```python
from build123d import *

# Parameters (mm, degrees)
F0_W      = 157
F0_H      = 90
F1_DEPTH  = 83
F3_DEPTH  = 90
F5_DEPTH  = 557
F6_R      = 22
F7_DEPTH  = 25
F7_FACE_R = 22
F8_DEPTH  = 185


with BuildPart() as f1:
    # F0 (on Top) → F1 (new body)
    with BuildSketch(Plane.XY):
        Rectangle(F0_W, F0_H)
    extrude(amount=F1_DEPTH)

    # F2 (on face) → F3 (join, through all)
    with BuildSketch(Plane.XZ.offset(45)):
        with BuildLine():
            Line((-78.5, 0), (-78.5, 83))
            ThreePointArc((-78.5, 83), (-89.175701, 41.5), (-78.5, 0))
        make_face()
        with BuildLine():
            ThreePointArc((78.5, 0), (89.175701, 41.5), (78.5, 83))
            Line((78.5, 83), (78.5, 0))
        make_face()
    extrude(amount=-F3_DEPTH)

    # F4 (on face) → F5 (cut)
    with BuildSketch(Plane.XZ.offset(45)):
        Polygon((-56.5, 0), (-4, 0), (48.5, 0), (48.5, 22), (-56.5, 22), align=None)
    extrude(amount=-F5_DEPTH, mode=Mode.SUBTRACT)

    # F6 (on face) → F7 (cut)
    with BuildSketch(Plane.XY.offset(83)):
        with BuildLine():
            ThreePointArc((0, -35), (24.748737, -24.748737), (35, 0))
            ThreePointArc((35, 0), (24.748737, 24.748737), (0, 35))
            ThreePointArc((0, 35), (-35, 0), (0, -35))
        make_face()
        Circle(F6_R, mode=Mode.SUBTRACT)
        with BuildLine():
            ThreePointArc((0, 35), (24.748737, 24.748737), (35, 0))
            ThreePointArc((35, 0), (24.748737, -24.748737), (0, -35))
            Line((0, -35), (78.5, -35))
            Line((78.5, -35), (78.5, 35))
            Line((78.5, 35), (0, 35))
        make_face()
        Polygon((93.384914, 35), (78.5, 35), (78.5, -35), (92.262775, -35), (93.384914, -35.542417), align=None)
    extrude(amount=-F7_DEPTH, mode=Mode.SUBTRACT)

    # F7_face (on face) → F8 (cut)
    with BuildSketch(Plane.XY.offset(83)):
        Circle(F7_FACE_R)
    extrude(amount=-F8_DEPTH, mode=Mode.SUBTRACT)


solid = f1.part
```
Geometry: final body of the model. Coordinates: model frame, mm. A direction names the side the tool comes from. Coordinates: 2 decimals unless noted, no trailing zeros. Order: outer loops, then holes, each group sorted by start corner. A loop starts at its lowest first (then second) coordinate and runs counter-clockwise, first axis right, second up. Notation, with made-up numbers: (69.25, 60.5) -> (87.25, 60.5) arc R27 ccw to (87.25, 96.5) -> close; hole circle Ø6 at (-21, -38.75). An arc over 180 degrees is marked (long way). Write item = value, one per line.
(1) Line query: line 1 (Y direction, x = 15, z = 66); line 2 (Y direction, x = 0, z = 47); line 3 (Z direction, x = -16.5, y = -20.5). Output: solid intervals per line, ascending.
Solved:
line_1 = -45 to -35, 35 to 45
line_2 = -45 to -22, 22 to 45
line_3 = 22 to 58
(2) Pin query (flat end, axial travel): pin 1 Ø5 at (x, y) = (21.5, -30.5) entering from +Z; pin 2 Ø8 at (y, z) = (29, 19) entering from -X; pin 3 Ø6.5 at (y, z) = (-5.5, 7.5) entering from +X. Return the tip coordinate at first contact, or that it passes through.
Solved:
pin_1 = 58
pin_2 = -87.16
pin_3 = 83.49
(3) Cut plane D-D on x = -2. Return loops of the section in (y, z).
Solved:
outline = (-45, 22) -> (-21.91, 22) -> (-21.91, 58) -> (-34.94, 58) -> (-34.94, 83) -> (-45, 83) -> close; (21.91, 22) -> (45, 22) -> (45, 83) -> (34.94, 83) -> (34.94, 58) -> (21.91, 58) -> close
(4) Cut plane C-C on x = 53.5. Return loops of the section in (y, z).
Solved:
outline = (-45, 0) -> (45, 0) -> (45, 83) -> (35, 83) -> (35, 58) -> (-35, 58) -> (-35, 83) -> (-45, 83) -> close
(5) Cut plane B-B on z = 10. Return loops of the section in (x, y).
Solved:
outline = (-83.2, -45) -> (-56.5, -45) -> (-56.5, 45) -> (-83.2, 45) -> close; (48.5, -45) -> (83.2, -45) -> (83.2, 45) -> (48.5, 45) -> close
(6) Access query for faces 5 (the flat face through (-15, -21, 22)), 6 (the flat face through (63, 1, 0)), 7 (the cylindrical face through (-34.99, 0.77, 70.68)). Directions: +Z, -Z, +X, -X, +Y, -Y. A direction counts if a zero-diameter tool reaches every point of the face in a straight line with its end or side. Return the directions, or none.
Solved:
face_5 = -Z, +Y, -Y
face_6 = -Z, +X, -X, +Y, -Y
face_7 = +Z, +X
(7) Cut plane A-A on y = 0. Return loops of the section in (x, z).
Solved:
outline = (-78.5, 0) -> (-56.5, 0) -> (-56.5, 22) -> (-22, 22) -> (-22, 58) -> (-35, 58) -> (-35, 83) -> (-78.5, 83) arc R86 ccw to start; (22, 22) -> (48.5, 22) -> (48.5, 0) -> (78.5, 0) arc R86 ccw to (87.58, 58) -> (22, 58) -> close
(8) Pull-direction query (Y, two-part tool) for faces 1 (the cylindrical face through (-4.769, -21.477, 40.252)), 2 (the flat face through (-68, 1, 0)), 3 (the flat face through (-1, -45, 42)), 4 (the flat face through (-1, 45, 42)); classes: pulls with the +Y half, pulls with the -Y half, needs draft (parallel to the pull), parting line crosses it, or undercut.
Solved:
face_1 = undercut
face_2 = needs draft
face_3 = pulls with the -Y half
face_4 = pulls with the +Y half
